CAD build for the part. Positions are in the model's coordinates, mm. Face numbers are marked on the shaded views. A direction names the side the tool comes from. Coordinates: 2 decimals unless noted, no trailing zeros. Write each loop counter-clockwise with the first axis right and the second up, starting at its lowest first coordinate (ties: lowest second). Pieces come first, ordered by that corner, then holes.
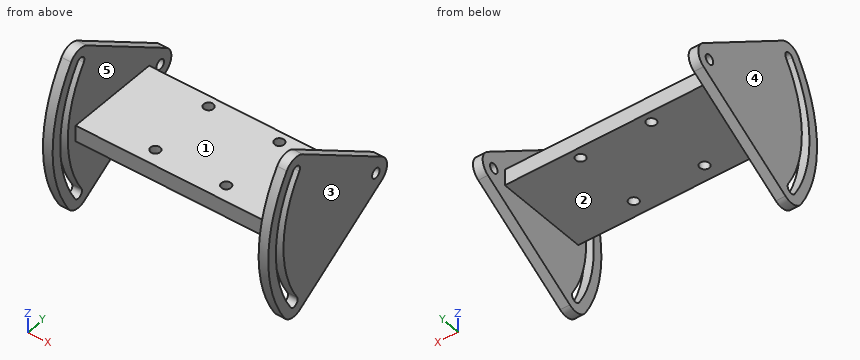
```python
from build123d import *

# Parameters (mm, degrees)
SKETCH_1_R               = 1.5
EXTRUDE_1_DEPTH          = 70
CUT_EXTRUDE_1_DEPTH      = 40
CUT_EXTRUDE_1_DEPTH_BACK = 48
SKETCH_3_W               = 64
SKETCH_3_H               = 30
SKETCH_4_R               = 1.5
CUT_EXTRUDE_2_DEPTH      = 10
CUT_EXTRUDE_4_DEPTH      = 17
CUT_EXTRUDE_4_DEPTH_BACK = 11
SKETCH_5_W               = 64
SKETCH_5_H               = 10
SKETCH_5_H_2             = 13


with BuildPart() as part:
    # 草图1 → 凸台-拉伸1 (new body)
    with BuildSketch(Plane(origin=(0, 0, 0), x_dir=(0, 0, -1), z_dir=(1, 0, 0))):
        with BuildLine():
            ThreePointArc((3.748616704, 13.830886654), (0.101280137, 15.922634297), (-3.638391548, 14.000830996))
            Line((-3.638391548, 14.000830996), (-25.044186814, -17.396344398))
            ThreePointArc((-25.044186814, -17.396344398), (-25.746563923, -20.773505291), (-23.851546095, -23.655771194))
            ThreePointArc((-23.851546095, -23.655771194), (-0.977489629, -30.968489282), (22.208659079, -24.715424983))
            ThreePointArc((22.208659079, -24.715424983), (24.234219774, -21.923355289), (23.687892423, -18.517466898))
            Line((23.687892423, -18.517466898), (3.748616704, 13.830886654))
        make_face()
        with BuildLine():
            ThreePointArc((20.640989027, -22.157611345), (-0.908490361, -27.96928287), (-22.167907547, -21.172756648))
            ThreePointArc((-22.167907547, -21.172756648), (-22.567595547, -19.0894301), (-20.484268999, -18.689742101))
            ThreePointArc((-20.484268999, -18.689742101), (-0.839491093, -24.970076458), (19.073318974, -19.599797708))
            ThreePointArc((19.073318974, -19.599797708), (21.136060819, -20.0948695), (20.640989027, -22.157611345))
        make_face(mode=Mode.SUBTRACT)
        with Locations((0, 11.52026822)):
            Circle(SKETCH_1_R, mode=Mode.SUBTRACT)
    extrude(amount=EXTRUDE_1_DEPTH)

    # 草图3 → 切除-拉伸1 (cut, two sides: drawn at the far end of the back side and taken through both)
    with BuildSketch(Plane(origin=(0, 0, 0), x_dir=(1, 0, 0), z_dir=(0, 1, 0)).offset(-CUT_EXTRUDE_1_DEPTH_BACK)):
        with Locations((35, 17.5)):
            Rectangle(SKETCH_3_W, SKETCH_3_H)
        with Locations((35, -17.5)):
            Rectangle(SKETCH_3_W, SKETCH_3_H)
    extrude(amount=CUT_EXTRUDE_1_DEPTH + CUT_EXTRUDE_1_DEPTH_BACK, mode=Mode.SUBTRACT)

    # 草图4 → 切除-拉伸2 (cut)
    with BuildSketch(Plane.XY.offset(2.5)):
        with Locations((24, 3.92379916)):
            Circle(SKETCH_4_R)
        with Locations((46, 3.92379916)):
            Circle(SKETCH_4_R)
        with Locations((46, -17.07620084)):
            Circle(SKETCH_4_R)
        with Locations((24, -17.07620084)):
            Circle(SKETCH_4_R)
    extrude(amount=-CUT_EXTRUDE_2_DEPTH, mode=Mode.SUBTRACT)

    # 草图5 → 切除-拉伸4 (cut, two sides: drawn at the far end of the back side and taken through both)
    with BuildSketch(Plane.XY.offset(2.5).offset(-CUT_EXTRUDE_4_DEPTH_BACK)):
        with Locations((35, -26.894014692)):
            Rectangle(SKETCH_5_W, SKETCH_5_H)
        with Locations((35, 13.645331632)):
            Rectangle(SKETCH_5_W, SKETCH_5_H_2)
    extrude(amount=CUT_EXTRUDE_4_DEPTH + CUT_EXTRUDE_4_DEPTH_BACK, mode=Mode.SUBTRACT)


solid = part.part
```
Item 1: Flat gauge pins, fed straight in: pin 1 Ø4 at (x, y) = (46, -17.08) entering from +Z; pin 2 Ø6 at (x, y) = (33.5, -7) entering from -Z; pin 3 Ø1.8 at (y, z) = (11.52, 0) entering from -X; pin 4 Ø1.5 at (x, z) = (24, 0.5) entering from +Y. Where does each tip first touch, or does it go through?
Item 2: Saw through at C-C, the plane y = -26. Write the cut outline in (x, z).
Item 3: Two-plate mould, pull along X, no slides. Class the marked faces 3, 4 and 5: +X half, -X half, draft (parallel to the pull), parting line (faces both ways), or undercut.
Item 4: Saw through at D-D, the plane z = 0. State how many separate pieces and enclosed holes the cut face has, and give its area (3 significant figures).
Item 5: Which spindle directions (+Z, -Z, +X, -X, +Y, -Y) get a long thin tool onto all of the face, cutting with end or side? Do the marked faces 1 and 2. Say none if no direction does.
Item 6: Wall check: line 1 along Y through (x, z) = (46, -1.3); line 2 along Y through (x, z) = (68, 0); line 3 along X through (y, z) = (-28.5, -8). Give the ranges that are in metal, low to high.
Item 7: Saw through at A-A, the plane x = 24. Write the cut outline in (y, z), and give its area (3 significant figures).
Item 8: Saw through at B-B, the plane z = -6.5. Write the cut outline in (x, y), and give its area (3 significant figures).
Working result:
1. pin 1: stops at z = 2.5
1. pin 2: stops at z = -2.5
1. pin 3: passes through
1. pin 4: stops at y = 7.15
2. outline: (0, -19.96) - (3, -19.96) - (3, -12.35) - (0, -12.35) - close; (0, 12.35) - (3, 12.35) - (3, 19.96) - (0, 19.96) - close; (67, -19.96) - (70, -19.96) - (70, -12.35) - (67, -12.35) - close; (67, 12.35) - (70, 12.35) - (70, 19.96) - (67, 19.96) - close
3. face 3: +X half
3. face 4: -X half
3. face 5: undercut
4. separate pieces: 5
4. enclosed holes: 4
4. area: 2,080 mm2
5. face 1: +Z, +Y, -Y
5. face 2: -Z, +Y, -Y
6. line 1: y = -21.89 to -18.58, -15.58 to 2.42, 5.42 to 7.15
6. line 2: y = -30.98 to -27.98, -24.98 to 10.02, 13.02 to 15.92
6. line 3: x = 0 to 3, 67 to 70
7. outline: (-21.89, -2.5) - (-18.58, -2.5) - (-18.58, 2.5) - (-21.89, 2.5) - close; (-15.58, -2.5) - (2.42, -2.5) - (2.42, 2.5) - (-15.58, 2.5) - close; (5.42, -2.5) - (7.15, -2.5) - (7.15, 2.5) - (5.42, 2.5) - close
7. area: 115 mm2
8. outline: (0, -30.48) - (3, -30.48) - (3, -27.44) - (0, -27.44) - close; (0, -24.4) - (3, -24.4) - (3, 9.37) - (0, 9.37) - close; (67, -30.48) - (70, -30.48) - (70, -27.44) - (67, -27.44) - close; (67, -24.4) - (70, -24.4) - (70, 9.37) - (67, 9.37) - close
8. area: 221 mm2
